Study the drawing (mm; zero at the part's minimum x, y, z) and answer. Round coordinates to 2 decimals unless told otherwise and drop trailing zeros. Write each loop counter-clockwise with the first axis right and the second up, starting at its lowest first coordinate (ties: lowest second). Pieces come first, ordered by that corner, then holes. Notation, with made-up numbers: (-39.5, -8.5) -> (-1.5, -8.5) arc R16 ccw to (-1.5, 4.5) -> close; hole circle Ø7 at (2, 2). An arc over 180 degrees is marked (long way). Return JSON: item names as keys, results as strings.
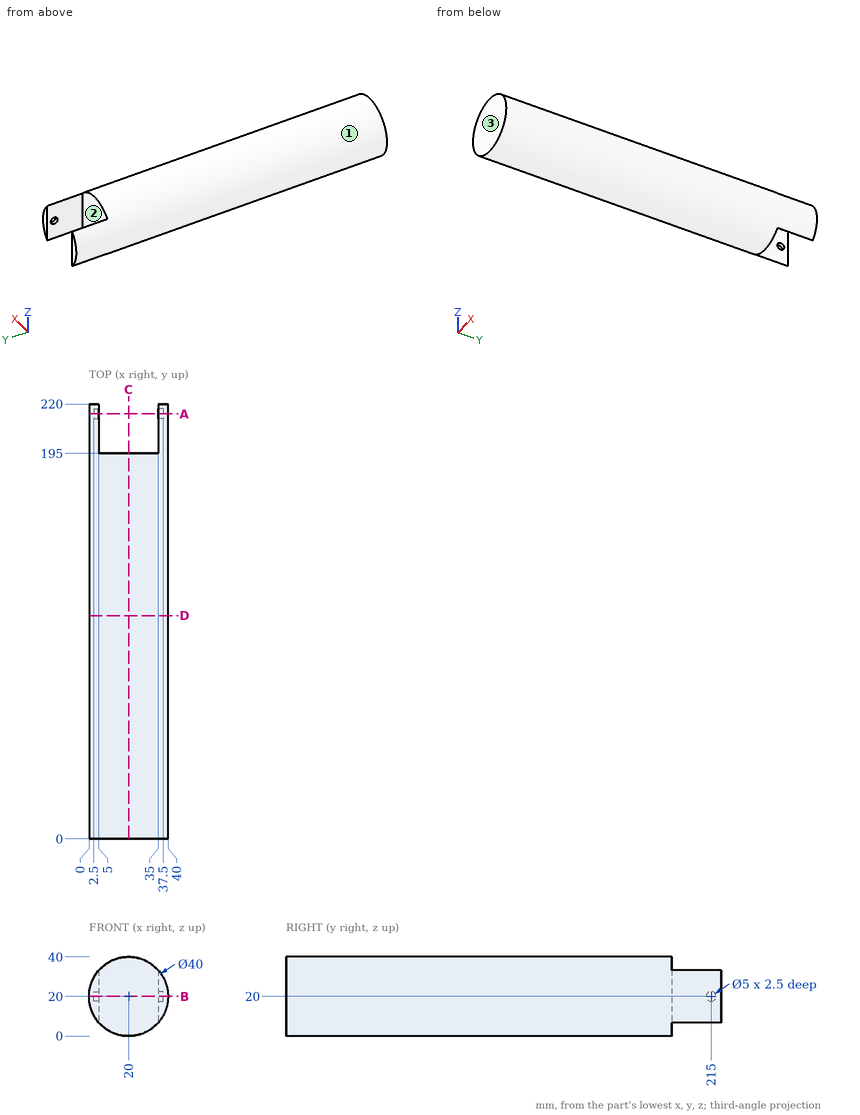
Item 1: Section C-C (x = 20) is taken. Give the vertices of the cut face in (y, z), then the cut area to 3 significant figures.
Worked answers:
{"outline": "(0, 0) -> (195, 0) -> (195, 40) -> (0, 40) -> close", "area": "7,800 mm2"}
Item 2: Straight lines are drawn through the part: L1, parallel to Y at x = 36.2, z = 20; L2, parallel to X at y = 196, z = 20; L3, parallel to Y at x = 11.5, z = 10. For each, find the intervals that lie inside material, in ascending order. Write a range as [from, to].
Worked answers:
{"L1": "y = [0, 212.5], [217.5, 220]", "L2": "x = [0, 5], [35, 40]", "L3": "y = [0, 195]"}
Item 3: Section D-D (y = 113) is taken. Give the vertices of the cut face in (x, z), then the cut area to 3 significant figures.
Worked answers:
{"outline": "circle Ø40 at (20, 20)", "area": "1,260 mm2"}
Item 4: For a pull along X with two mould halves and no side action, classify the marked faces 1, 2 and 3 as released by +X, released by -X, zero draft, split by the parting line, or undercut.
Worked answers:
{"face 1": "split by the parting line", "face 2": "undercut", "face 3": "zero draft"}
Item 5: Section A-A (y = 215) is taken. Give the vertices of the cut face in (x, z), then the cut area to 3 significant figures.
Worked answers:
{"outline": "(2.5, 17.5) -> (2.5, 22.5) -> (5, 22.5) -> (5, 33.23) arc R20 ccw to (5, 6.77) -> (5, 17.5) -> close; (35, 6.77) arc R20 ccw to (35, 33.23) -> (35, 22.5) -> (37.5, 22.5) -> (37.5, 17.5) -> (35, 17.5) -> close", "area": "156 mm2"}
Item 6: Flat-ended cylindrical pins translate along their axes: pin 1 (4 mm diameter, centred on x = 34.5, y = 120, fed in from -Z); pin 2 (10 mm diameter, centred on x = 23.5, y = 100.5, fed in from +Z); pin 3 (20 mm diameter, centred on y = 203.5, z = 13.5, fed in from +X); pin 4 (7.5 mm diameter, centred on y = 202.5, z = 15, fed in from -X). Find the tip coordinate at first contact, or state that the pin passes through.
Worked answers:
{"pin 1": "stops at z = 4.39", "pin 2": "stops at z = 40", "pin 3": "stops at x = 40", "pin 4": "stops at x = 0.04"}
Item 7: Section B-B (z = 20) is taken. Give the vertices of the cut face in (x, y).
Worked answers:
{"outline": "(0, 0) -> (40, 0) -> (40, 220) -> (35, 220) -> (35, 217.5) -> (37.5, 217.5) -> (37.5, 212.5) -> (35, 212.5) -> (35, 195) -> (5, 195) -> (5, 212.5) -> (2.5, 212.5) -> (2.5, 217.5) -> (5, 217.5) -> (5, 220) -> (0, 220) -> close"}
